from build123d import *

# Parameters (mm, degrees)
F0_W     = 132.481672
F0_H     = 84.847815
F1_DEPTH = 83.058
F2_W     = 35.940319
F2_H     = 24.245456
F4_DEPTH = 80.772
F3_W     = 45.638506
F3_H     = 23.389732
F5_DEPTH = 82.296
F6_R     = 32.500143


with BuildPart() as f1:
    # F0 (on Top) → F1 (new body)
    with BuildSketch(Plane.XY):
        with Locations((3.225211, -2.604976)):
            Rectangle(F0_W, F0_H)
    extrude(amount=F1_DEPTH)

    # F2 (on face) → F4 (cut)
    with BuildSketch(Plane.XY.offset(83.058)):
        with Locations((-39.363209, 19.396365)):
            Rectangle(F2_W, F2_H)
    extrude(amount=-F4_DEPTH, mode=Mode.SUBTRACT)

    # F3 (on face) → F5 (cut)
    with BuildSketch(Plane.XY.offset(83.058)):
        with Locations((35.369841, 19.253743)):
            Rectangle(F3_W, F3_H)
    extrude(amount=-F5_DEPTH, mode=Mode.SUBTRACT)

    # F6
    f6_edges = [f1.edges().sort_by_distance(p)[0] for p in [
        (3.225211, -45.028884, 83.058),
    ]]
    fillet(f6_edges, radius=F6_R)


solid = f1.part
Input: part model. Units: mm. Frame: model coordinates. A direction names the side the tool comes from. Coordinates: 2 decimals unless noted, no trailing zeros. Loops run counter-clockwise (first coordinate to the right, second up) from the corner with the lowest first, then second, coordinate; pieces in that order, holes last.
(1) Material intervals for probe 1 along X at (y, z) = (29, 19); probe 2 along Y at (x, z) = (-31, 4); probe 3 along Y at (x, z) = (54.5, 6), sorted ascending.
(2) Section D-D on x = 2.5. Return the cut outline in (y, z).
(3) Pull-direction query (X, two-part tool) for faces 3 (the face through (2, -2, 0)), 4 (the face through (69.466, -3, 41)), 5 (the face through (58.189, 19, 42)); classes: released by +X, released by -X, zero draft, split by the parting line, or undercut.
(4) Section A-A on z = 31.5. Return the cut outline in (x, y).
(5) Set-up query: faces 1 (the face through (-63.016, -3, 41)), 2 (the face through (35, 19, 0.762)). Return all of +Z, -Z, +X, -X, +Y, -Y with unobstructed straight access to the full face (end or side cutting, diameter ignored); none if empty.
(6) Section B-B on x = 53. Return the cut outline in (y, z).
(7) First-contact query: pin 1 Ø11.5 at (x, y) = (34, 24.5) entering from +Z; pin 2 Ø1.5 at (x, z) = (-24, 73.5) entering from -Y; pin 3 Ø10 at (x, y) = (20, -31.5) entering from +Z. Flat tips, straight axial feed; report the tip coordinate or a pass-through.
(8) Section C-C on y = 13. Return the cut outline in (x, z).
Data:
1. probe 1: x = -63.02 to -57.33, -21.39 to 12.55, 58.19 to 69.47
1. probe 2: y = -45.03 to 7.27, 31.52 to 39.82
1. probe 3: y = -45.03 to 7.56, 30.95 to 39.82
2. outline: (-45.03, 0) - (39.82, 0) - (39.82, 83.06) - (-12.53, 83.06) arc R32.5 ccw to (-45.03, 50.56) - close
3. face 3: zero draft
3. face 4: released by +X
3. face 5: undercut
4. outline: (-63.02, -45.03) - (69.47, -45.03) - (69.47, 39.82) - (-63.02, 39.82) - close; hole (-57.33, 7.27) - (-21.39, 7.27) - (-21.39, 31.52) - (-57.33, 31.52) - close; hole (12.55, 7.56) - (58.19, 7.56) - (58.19, 30.95) - (12.55, 30.95) - close
5. face 1: +Z, -Z, -X, +Y, -Y
5. face 2: +Z
6. outline: (-45.03, 0) - (39.82, 0) - (39.82, 83.06) - (30.95, 83.06) - (30.95, 0.76) - (7.56, 0.76) - (7.56, 83.06) - (-12.53, 83.06) arc R32.5 ccw to (-45.03, 50.56) - close
7. pin 1: stops at z = 0.76
7. pin 2: stops at y = -36.27
7. pin 3: stops at z = 79.9
8. outline: (-63.02, 0) - (69.47, 0) - (69.47, 83.06) - (58.19, 83.06) - (58.19, 0.76) - (12.55, 0.76) - (12.55, 83.06) - (-21.39, 83.06) - (-21.39, 2.29) - (-57.33, 2.29) - (-57.33, 83.06) - (-63.02, 83.06) - close
